from build123d import *

# Parameters (mm, degrees)
BASESKETCH1_R             = 12
BASESKETCH1_R_2           = 1.55
WIDTHBOSS_EXTRUDE1_DEPTH  = 3
SKETCH2_W                 = 50
SKETCH2_H                 = 3
HEIGHTBOSS_EXTRUDE2_DEPTH = 50
SLOTSCUT_EXTRUDE1_DEPTH   = 87.706401148
WEDGESKETCH4_W            = 3
WEDGESKETCH4_H            = 20
ANGLEBOSS_EXTRUDE3_DEPTH  = 20
CHAMFER1_SIZE             = 20


with BuildPart() as part:
    # BaseSketch1 → WidthBoss-Extrude1 (new body)
    with BuildSketch(Plane(origin=(0, 0, 0), x_dir=(1, 0, 0), z_dir=(0, 1, 0))):
        Polygon((0, 0), (50, 0), (50, 46.99479618), (46.99479618, 50), (3.00520382, 50), (0, 46.99479618), align=None)
        with Locations(Location((25, 30, 0), (0, 0, 270))):
            Circle(BASESKETCH1_R, mode=Mode.SUBTRACT)
        with Locations(Location((9.5, 45.5, 0), (0, 0, 270))):
            Circle(BASESKETCH1_R_2, mode=Mode.SUBTRACT)
        with Locations(Location((40.5, 45.5, 0), (0, 0, 270))):
            Circle(BASESKETCH1_R_2, mode=Mode.SUBTRACT)
        with Locations(Location((40.5, 14.5, 0), (0, 0, 270))):
            Circle(BASESKETCH1_R_2, mode=Mode.SUBTRACT)
        with Locations(Location((9.5, 14.5, 0), (0, 0, 270))):
            Circle(BASESKETCH1_R_2, mode=Mode.SUBTRACT)
    extrude(amount=WIDTHBOSS_EXTRUDE1_DEPTH)

    # Sketch2 → HeightBoss-Extrude2 (add)
    with BuildSketch(Plane(origin=(0, 3, 0), x_dir=(1, 0, 0), z_dir=(0, 1, 0))):
        with Locations((25, 1.5)):
            Rectangle(SKETCH2_W, SKETCH2_H)
    extrude(amount=HEIGHTBOSS_EXTRUDE2_DEPTH)

    # Sketch3 → SlotsCut-Extrude1 (cut, through all)
    with BuildSketch(Plane(origin=(0, 0, -3), x_dir=(-1, 0, 0), z_dir=(0, 0, -1))):
        with BuildLine():
            Line((-42.6, 14.3), (-42.6, 43.9))
            ThreePointArc((-42.6, 43.9), (-40.5, 46), (-38.4, 43.9))
            Line((-38.4, 43.9), (-38.4, 14.3))
            ThreePointArc((-38.4, 14.3), (-40.5, 12.2), (-42.6, 14.3))
        make_face()
        with BuildLine():
            Line((-11.6, 14.3), (-11.6, 43.9))
            ThreePointArc((-11.6, 43.9), (-9.5, 46), (-7.4, 43.9))
            Line((-7.4, 43.9), (-7.4, 14.3))
            ThreePointArc((-7.4, 14.3), (-9.5, 12.2), (-11.6, 14.3))
        make_face()
    extrude(amount=-SLOTSCUT_EXTRUDE1_DEPTH, mode=Mode.SUBTRACT)

    # WedgeSketch4 → AngleBoss-Extrude3 (add)
    with BuildSketch(Plane(origin=(0, 3, 0), x_dir=(1, 0, 0), z_dir=(0, 1, 0))):
        with Locations((48.5, 13)):
            Rectangle(WEDGESKETCH4_W, WEDGESKETCH4_H)
        with Locations((1.5, 13)):
            Rectangle(WEDGESKETCH4_W, WEDGESKETCH4_H)
    extrude(amount=ANGLEBOSS_EXTRUDE3_DEPTH)

    # Chamfer1
    chamfer1_edges = [part.edges().sort_by_distance(p)[0] for p in [
        (48.5, 23, -23),
        (1.5, 23, -23),
    ]]
    chamfer(chamfer1_edges, length=CHAMFER1_SIZE - 0.0001)  # a hair under: the kernel refuses the full size


solid = part.part
Verification items for the finished model (mm, model axes). A direction names the side the tool comes from. Give positions to 0.01 mm unless a question says otherwise; leave off trailing zeros. Loops run counter-clockwise (first coordinate to the right, second up) from the corner with the lowest first, then second, coordinate; pieces in that order, holes last. Notation, with made-up numbers: (21.5, 80.25) - (33.5, 80.25) arc R7 cw to (33.5, 84.25) - close; hole circle Ø7 at (3.5, 43.5). An arc over 180 degrees is marked (long way). Write item = value, one per line. Start each with the question number.
Q1. Mould release check, pull along Z, two halves, no side actions. Record for faces 4 (the face through (9.57, 1.48, -16.05)), 5 (the face through (50, 13, -11)), 6 (the face through (48.518, 1.479, -48.476)): released by +Z, released by -Z, zero draft, split by the parting line, or undercut.
Q2. Depth check by flat-ended pin: P1, Ø8, axis at x = 13, z = -17.5, coming from the +Y side; P2, Ø8, axis at x = 17, y = 40, coming from the -Z side. Enter the tip coordinate at first touch or a pass-through.
Q3. Cross-section at A-A, the plane x = 9.5. Enter the section's corners in (y, z).
Q4. Cross-section at D-D, the plane x = 35. Enter the section's corners in (y, z), and give its area (3 significant figures).
Q5. Tool access check on faces 1 (the face through (39.56, 1.48, -15.73)), 2 (the face through (40.5, 46, -1.5)), 3 (the face through (25, 3, -16)). Record the directions out of +Z, -Z, +X, -X, +Y, -Y that give a thin tool (end or side, any length) a straight path to the whole face; none if there is none.
Q6. Cross-section at C-C, the plane z = -14.5. Enter the section's corners in (x, y).
Q7. Cross-section at B-B, the plane y = 25. Enter the section's corners in (x, z).
Q8. Thickness scan on line 1 (X direction, y = 1.5, z = -45.5); line 2 (Z direction, x = 9, y = 2); line 3 (Z direction, x = 4, y = 12.5). Record the ranges inside material, lowest first.
Answer key:
q1.face_4 = undercut
q1.face_5 = zero draft
q1.face_6 = released by -Z
q2.P1 = 3
q2.P2 = -3
q3.outline = (0, -50) - (3, -50) - (3, -47.05) - (0, -47.05) - close; (0, -43.95) - (3, -43.95) - (3, -16.05) - (0, -16.05) - close; (0, -12.95) - (3, -12.95) - (3, -3) - (12.2, -3) - (12.2, 0) - (0, 0) - close; (46, -3) - (53, -3) - (53, 0) - (46, 0) - close
q4.outline = (0, -50) - (3, -50) - (3, -36.63) - (0, -36.63) - close; (0, -23.37) - (3, -23.37) - (3, -3) - (53, -3) - (53, 0) - (0, 0) - close
q4.area = 260 mm^2
q5.face_1 = +Y, -Y
q5.face_2 = +Z, -Z
q5.face_3 = -Z, +Y
q6.outline = (0, 0) - (7.95, 0) - (7.95, 3) - (3, 3) - (3, 11.5) - (0, 11.5) - close; (11.05, 0) - (38.95, 0) - (38.95, 3) - (11.05, 3) - close; (42.05, 0) - (50, 0) - (50, 11.5) - (47, 11.5) - (47, 3) - (42.05, 3) - close
q7.outline = (0, -3) - (7.4, -3) - (7.4, 0) - (0, 0) - close; (11.6, -3) - (38.4, -3) - (38.4, 0) - (11.6, 0) - close; (42.6, -3) - (50, -3) - (50, 0) - (42.6, 0) - close
q8.line_1 = 0 to 7.95, 11.05 to 38.95, 42.05 to 50
q8.line_2 = -50 to -46.97, -44.03 to -15.97, -13.03 to 0
q8.line_3 = -3 to 0
